Read the model definition and answer for the solid it produces. Units are mm, in the model's axes. A direction names the side the tool comes from. Coordinates: 2 decimals unless noted, no trailing zeros. Order: outer loops, then holes, each group sorted by start corner. A loop starts at its lowest first (then second) coordinate and runs counter-clockwise, first axis right, second up. Notation, with made-up numbers: (-37.5, 36.25) -> (-5.5, 36.25) arc R13 ccw to (-5.5, 61.25) -> close; hole circle Ø9 at (-17, 39.25). An arc over 180 degrees is marked (long way). Answer as a JSON object with one key per item and string values. Group by question number.
1) Consider L1, parallel to Z at x = -3, y = 9; L2, parallel to Y at x = 6.5, z = 1; L3, parallel to Y at x = -19, z = -7. Determine where each line is inside the solid, lowest interval first.
2) Determine the mould class of faces 6 (the flat face through (-45, -8, 40.636)), 7 (the flat face through (-16, -7.036, -1)), 8 (the flat face through (-33.98, -5.99, -110.41)) for opening direction X: released by +X, released by -X, zero draft, split by the parting line, or undercut.
3) Given pin 1 (16.5 mm diameter, centred on x = -17.5, z = -172.5, fed in from +Y); pin 2 (16.5 mm diameter, centred on x = -17, z = 8.5, fed in from +Y); pin 3 (8 mm diameter, centred on y = 1, z = -52, fed in from +X), each flat-ended and moving along its own axis, determine where each tip first touches the part or whether it passes through.
4) Section C-C on x = -36 is taken. Determine the outline of the cut face in (y, z), and give its area (3 significant figures).
5) Section D-D on z = -52 is taken. Determine the outline of the cut face in (x, y).
6) A tool of negligible diameter and unlimited length cuts with its end or side. For faces 1 (the flat face through (-33.74, -5.99, -26.66)), 2 (the flat face through (8, 16.964, -1)), 3 (the flat face through (-43, -7, -172)), 4 (the flat face through (-16, -7.036, -168)), 5 (the flat face through (-29.991, -5.496, 25.517)), from which of +Z, -Z, +X, -X, +Y, -Y can it reach the whole face along a straight path? Write none if from no direction.
7) Section B-B on z = -183 is taken. Determine the outline of the cut face in (x, y).
8) Section A-A on x = -14.5 is taken. Determine the outline of the cut face in (y, z).
from build123d import *

# Parameters (mm, degrees)
SKETCH_1_W          = 250
SKETCH_1_H          = 4
EXTRUDE_1_DEPTH     = 20
EXTRUDE_1_2_DEPTH   = 20
SKETCH_2_W          = 250
SKETCH_2_H          = 28
EXTRUDE_2_DEPTH     = 4
SKETCH_3_W          = 250
SKETCH_3_H          = 4
EXTRUDE_3_DEPTH     = 51
EXTRUDE_4_DEPTH     = 250
CUT_EXTRUDE_1_DEPTH = 55
FILLET_1_R          = 2
CUT_EXTRUDE_2_DEPTH = 250


with BuildPart() as part:
    # Sketch 1 → Extrude 1 (new body)
    with BuildSketch(Plane(origin=(0, 0, 0), x_dir=(0, 0, -1), z_dir=(1, 0, 0))):
        with Locations((84.36416185, 14.963552055)):
            Rectangle(SKETCH_1_W, SKETCH_1_H)
    extrude(amount=EXTRUDE_1_DEPTH)



with BuildPart() as body_2:
    # Sketch 1 → Extrude 1 2 (new body)
    with BuildSketch(Plane(origin=(0, 0, 0), x_dir=(0, 0, -1), z_dir=(1, 0, 0))):
        with Locations((84.36416185, -9.036447945)):
            Rectangle(SKETCH_1_W, SKETCH_1_H)
    extrude(amount=EXTRUDE_1_2_DEPTH)


with BuildPart() as part_1:
    add(part.part)

    add(body_2.part)  # Extrude 2 merges body 2
    # Sketch 2 → Extrude 2 (add)
    with BuildSketch(Plane.ZY):
        with Locations((-84.36416185, 2.963552055)):
            Rectangle(SKETCH_2_W, SKETCH_2_H)
    extrude(amount=EXTRUDE_2_DEPTH)

    # Sketch 3 → Extrude 3 (add)
    with BuildSketch(Plane.ZY.offset(4)):
        with Locations((-84.36416185, -9.036447945)):
            Rectangle(SKETCH_3_W, SKETCH_3_H)
    extrude(amount=EXTRUDE_3_DEPTH)

    # Sketch 5 → Extrude 4 (add)
    with BuildSketch(Plane.XY.offset(40.63583815)):
        Polygon((-4, -7.036447945), (-55, -7.036447945), (-4, 7.963552055), align=None)
    extrude(amount=-EXTRUDE_4_DEPTH)

    # Sketch 7 → Cut-Extrude 1 (cut)
    with BuildSketch(Plane(origin=(0, 16.963552055, 0), x_dir=(1, 0, 0), z_dir=(0, 1, 0))):
        Polygon((-38.720043801, 209.36416185), (-20.437285277, 177.697495183), (20, 177.697495183), (20, 209.36416185), align=None)
        Polygon((20, 157.697495183), (-24.717241476, 157.697495183), (-43, 126.030828516), (-24.717241476, 94.36416185), (20, 94.36416185), align=None)
        Polygon((-43, 196.77726344), (-43, 146.030828516), (-28.350766068, 171.404045978), align=None)
        Polygon((-43, 106.030828516), (-30.490744168, 84.36416185), (-43, 84.36416185), align=None)
    cut_extrude_1 = extrude(amount=-CUT_EXTRUDE_1_DEPTH, mode=Mode.SUBTRACT)

    # Mirror 1: Cut-Extrude 1 across plane
    add(cut_extrude_1.mirror(Plane(origin=(0, 0, -84.36416185), x_dir=(1, 0, 0), z_dir=(0, 0, -1))), mode=Mode.SUBTRACT)

    # Fillet 1
    fillet_1_edges = [part_1.edges().sort_by_distance(p)[0] for p in [
        (-24.717241476, -4.583101103, -94.36416185),
        (-43, -7.271742062, -126.030828516),
        (-24.717241476, -4.583101103, -157.697495183),
        (-43, -7.271742062, -106.030828516),
        (-30.490744168, -5.432145617, -84.36416185),
        (-20.437285277, -3.95369578, -177.697495183),
        (-28.350766068, -5.117442955, 2.675722279),
        (-43, -7.271742062, 28.048939741),
        (-43, -7.271742062, -22.697495183),
        (-24.717241476, -4.583101103, -11.030828516),
        (-43, -7.271742062, -42.697495183),
        (-24.717241476, -4.583101103, -74.36416185),
        (-43, -7.271742062, -62.697495183),
        (-20.437285277, -3.95369578, 8.969171484),
        (-43, -7.271742062, -196.77726344),
        (-28.350766068, -5.117442955, -171.404045978),
        (-43, -7.271742062, -146.030828516),
    ]]
    fillet(fillet_1_edges, radius=FILLET_1_R)

    # Sketch 8 → Cut-Extrude 2 (cut)
    with BuildSketch(Plane(origin=(0, 0, -209.36416185), x_dir=(-1, 0, 0), z_dir=(0, 0, -1))):
        with BuildLine():
            Line((4, 1.12118318), (4, -5.036447945))
            ThreePointArc((4, -5.036447945), (4.585786438, -6.450661507), (6, -7.036447945))
            Line((6, -7.036447945), (26.935945824, -7.036447945))
            ThreePointArc((26.935945824, -7.036447945), (28.915524315, -5.321525122), (27.500278472, -3.117716942))
            Line((27.500278472, -3.117716942), (6.564332648, 3.039914183))
            ThreePointArc((6.564332648, 3.039914183), (4.80180663, 2.72253656), (4, 1.12118318))
        make_face()
    extrude(amount=-CUT_EXTRUDE_2_DEPTH, mode=Mode.SUBTRACT)


solid = part_1.part
Worked answers:
{
 "1": {"L1": "z = -177.7 to -157.7, -94.36 to -74.36, -11.03 to 8.97", "L2": "y = -11.04 to -7.04, 12.96 to 16.96", "L3": "y = -11.04 to -7.04, -0.62 to 3.55"},
 "2": {"face 6": "zero draft", "face 7": "undercut", "face 8": "released by +X"},
 "3": {"pin 1": "stops at y = 6.42", "pin 2": "stops at y = 6.57", "pin 3": "stops at x = -35.77"},
 "4": {"outline": "(-11.04, -204.65) -> (-1.45, -204.65) -> (-1.45, -184.65) -> (-11.04, -184.65) -> close; (-11.04, -158.16) -> (-1.45, -158.16) -> (-1.45, -138.16) -> (-11.04, -138.16) -> close; (-11.04, -113.91) -> (-1.45, -113.91) -> (-1.45, -93.91) -> (-11.04, -93.91) -> close; (-11.04, -74.82) -> (-1.45, -74.82) -> (-1.45, -54.82) -> (-11.04, -54.82) -> close; (-11.04, -30.57) -> (-1.45, -30.57) -> (-1.45, -10.57) -> (-11.04, -10.57) -> close; (-11.04, 15.92) -> (-1.45, 15.92) -> (-1.45, 35.92) -> (-11.04, 35.92) -> close", "area": "1,150 mm²"},
 "5": {"outline": "(-55, -11.04) -> (-37.63, -11.04) -> (-37.63, -1.93) -> (-55, -7.04) -> close"},
 "6": {"face 1": "+X, +Y, -Y", "face 2": "+Z, -Z, +X, -X, +Y", "face 3": "+Y, -Y", "face 4": "+Z, -Z", "face 5": "+Z, +X, +Y, -Y"},
 "7": {"outline": "(-55, -11.04) -> (-43, -11.04) -> (-43, -3.51) -> (-55, -7.04) -> close; (-35.05, -11.04) -> (-23.5, -11.04) -> (-23.5, -7.04) -> (-26.94, -7.04) arc R2 cw to (-27.5, -3.12) -> (-23.5, -1.94) -> (-23.5, 2.23) -> (-35.05, -1.17) -> close"},
 "8": {"outline": "(-11.04, -177.7) -> (-7.04, -177.7) -> (-7.04, -157.7) -> (-11.04, -157.7) -> close; (-11.04, -94.36) -> (-7.04, -94.36) -> (-7.04, -74.36) -> (-11.04, -74.36) -> close; (-11.04, -11.03) -> (-7.04, -11.03) -> (-7.04, 8.97) -> (-11.04, 8.97) -> close; (0.71, -177.7) -> (4.88, -177.7) -> (4.88, -157.7) -> (0.71, -157.7) -> close; (0.71, -94.36) -> (4.88, -94.36) -> (4.88, -74.36) -> (0.71, -74.36) -> close; (0.71, -11.03) -> (4.88, -11.03) -> (4.88, 8.97) -> (0.71, 8.97) -> close"}
}
